Check sheet for the modelled part. Datum: model origin and axes. Units: mm. A direction names the side the tool comes from. Give positions to 0.01 mm unless a question says otherwise; leave off trailing zeros. Write each loop counter-clockwise with the first axis right and the second up, starting at its lowest first coordinate (ties: lowest second). Pieces come first, ordered by that corner, then holes. Notation, with made-up numbers: (29.5, -29.5) -> (70.5, -29.5) arc R16 cw to (70.5, -5.5) -> close; hole circle Ø8 at (36.5, 77.25). An arc over 180 degrees is marked (long way). Use a Markdown table: item, result. Add a question column.
1. Set-up check for faces 4 (the flat face through (24.195, 6, 4)), 5 (the flat face through (30.48, 93, 4)), 6 (the cylindrical face through (46.492, 44.249, 3.757)), 7 (the flat face through (78, 89.408, 4)): record each of +Z, -Z, +X, -X, +Y, -Y from which the full face is reachable in a straight line by a thin tool's end or side.
2. Cross-section at B-B (y = 12.7). Enter the section's corners in (x, z).
3. Scan lines: probe 1 along Z at (x, y) = (7.5, 24); probe 2 along X at (y, z) = (78, 6.5); probe 3 along X at (y, z) = (57.5, 4.75). Record each from-to range of solid material in increasing order. Write a range as [from, to].
4. Cross-section at A-A (x = 17). Enter the section's corners in (y, z).
5. Cross-section at D-D (x = 61). Enter the section's corners in (y, z), then the cut area to 3 significant figures.
6. Release check for a two-part mould opening along Z. For faces 1 (the cylindrical face through (10.454, 12.799, 1.252)), 2 (the flat face through (9, 45, 5.08)), 3 (the flat face through (54, 71, 5.08)) record: released by +Z, released by -Z, zero draft, split by the parting line, or undercut.
7. Gauge pin test, flat ends, axial feed: P1, Ø1.9, axis at y = 93, z = 4, coming from the +X side; P2, Ø3, axis at x = 67.5, y = 88.5, coming from the -Z side; P3, Ø1.9, axis at x = 36.51, y = 89.09, coming from the -Z side. Record the tip position at first contact, or that the pin passes through.
8. Cross-section at C-C (z = 3.75). Count the separate pieces of the cut face and the enclosed holes in it, then the cut area to 3 significant figures.
from build123d import *

# Parameters (mm, degrees)
F0_R     = 2.2479
F0_R_2   = 3.175
F0_R_3   = 11.43
F0_R_4   = 2.8575
F1_DEPTH = 2.54
F2_R     = 2.2479
F2_R_2   = 3.175
F2_R_3   = 2.8575
F2_R_4   = 1.574685516
F3_DEPTH = 2.54
F4_R     = 2.2479
F4_R_2   = 1.574685516
F4_R_3   = 11.4450762602
F5_DEPTH = 2.54
F6_DEPTH = 5.08
F7_W     = 22.86
F7_H     = 2.54
F8_DEPTH = 89.409


with BuildPart() as f1:
    # F0 (on Top) → F1 (new body)
    with BuildSketch(Plane.XY):
        Polygon((0, 89.408), (0, 0), (24.1954457015, 0), (24.1954457015, 11.3160238358), (82.55, 38.608), (82.55, 89.408), (73.66, 89.408), (73.66, 95.758), (30.48, 95.758), (30.48, 89.408), align=None)
        with Locations((12.7, 12.7)):
            Circle(F0_R, mode=Mode.SUBTRACT)
        with Locations((12.7, 44.704)):
            Circle(F0_R, mode=Mode.SUBTRACT)
        with Locations((45.4550236464, 46.2430119514)):
            Circle(F0_R, mode=Mode.SUBTRACT)
        with Locations((36.5125, 57.9755)):
            Circle(F0_R_2, mode=Mode.SUBTRACT)
        with Locations((12.7, 76.708)):
            Circle(F0_R, mode=Mode.SUBTRACT)
        with Locations((36.5125, 89.0905)):
            Circle(F0_R_2, mode=Mode.SUBTRACT)
        with Locations((67.6275, 57.9755)):
            Circle(F0_R_2, mode=Mode.SUBTRACT)
        with Locations((76.7535641789, 48.0743087828)):
            Circle(F0_R, mode=Mode.SUBTRACT)
        with Locations((52.07, 73.533)):
            Circle(F0_R_3, mode=Mode.SUBTRACT)
        with Locations((78.0854150653, 76.0432183743)):
            Circle(F0_R, mode=Mode.SUBTRACT)
        with Locations((67.6275, 89.0905)):
            Circle(F0_R_2, mode=Mode.SUBTRACT)
        with Locations((52.07, 73.533)):
            Circle(F0_R_3)
        with Locations((52.07, 73.533)):
            Circle(F0_R_4, mode=Mode.SUBTRACT)
    extrude(amount=F1_DEPTH)

    # F2 (on face) → F3 (join)
    with BuildSketch(Plane.XY.offset(2.54)):
        Polygon((30.48, 89.408), (25.4, 89.408), (25.4, 11.8793846154), (82.55, 38.608), (82.55, 89.408), (73.66, 89.408), (73.66, 95.758), (30.48, 95.758), align=None)
        with Locations((45.4550236464, 46.2430119514)):
            Circle(F2_R, mode=Mode.SUBTRACT)
        with Locations((36.5125, 57.9755)):
            Circle(F2_R_2, mode=Mode.SUBTRACT)
        with Locations((36.5125, 89.0905)):
            Circle(F2_R_2, mode=Mode.SUBTRACT)
        with Locations((67.6275, 57.9755)):
            Circle(F2_R_2, mode=Mode.SUBTRACT)
        with Locations((76.7535641789, 48.0743087828)):
            Circle(F2_R, mode=Mode.SUBTRACT)
        with Locations((52.07, 73.533)):
            Circle(F2_R_3, mode=Mode.SUBTRACT)
        with Locations((78.0854150653, 76.0432183743)):
            Circle(F2_R, mode=Mode.SUBTRACT)
        with Locations((67.6275, 89.0905)):
            Circle(F2_R_2, mode=Mode.SUBTRACT)
        with Locations((36.5125, 57.9755)):
            Circle(F2_R_2)
        with Locations((36.5125, 57.9755)):
            Circle(F2_R_4, mode=Mode.SUBTRACT)
        with Locations((67.6275, 57.9755)):
            Circle(F2_R_2)
        with Locations((67.6275, 57.9755)):
            Circle(F2_R_4, mode=Mode.SUBTRACT)
        with Locations((67.6275, 89.0905)):
            Circle(F2_R_2)
        with Locations((67.6275, 89.0905)):
            Circle(F2_R_4, mode=Mode.SUBTRACT)
        with Locations((36.5125, 89.0905)):
            Circle(F2_R_2)
        with Locations((36.5125, 89.0905)):
            Circle(F2_R_4, mode=Mode.SUBTRACT)
    extrude(amount=F3_DEPTH)

    # F4 (on face) → F5 (join)
    with BuildSketch(Plane.XY.offset(5.08)):
        Polygon((30.48, 89.408), (25.4, 89.408), (25.4, 11.8793846154), (82.55, 38.608), (82.55, 89.408), (73.66, 89.408), (73.66, 95.758), (30.48, 95.758), align=None)
        with Locations((45.4550236464, 46.2430119514)):
            Circle(F4_R, mode=Mode.SUBTRACT)
        with Locations((36.5125, 57.9755)):
            Circle(F4_R_2, mode=Mode.SUBTRACT)
        with Locations((36.5125, 89.0905)):
            Circle(F4_R_2, mode=Mode.SUBTRACT)
        with Locations((67.6275, 57.9755)):
            Circle(F4_R_2, mode=Mode.SUBTRACT)
        with Locations((76.7535641789, 48.0743087828)):
            Circle(F4_R, mode=Mode.SUBTRACT)
        with Locations((52.07, 73.533)):
            Circle(F4_R_3, mode=Mode.SUBTRACT)
        with Locations((78.0854150653, 76.0432183743)):
            Circle(F4_R, mode=Mode.SUBTRACT)
        with Locations((67.6275, 89.0905)):
            Circle(F4_R_2, mode=Mode.SUBTRACT)
    extrude(amount=F5_DEPTH)

    # F6 (add): a face of the model
    f6_faces = [f1.faces().sort_by_distance(p)[0] for p in [
        (12.7, 88.4785404547, 2.54),
    ]]
    extrude(f6_faces, amount=F6_DEPTH)

    # F7 (on face) → F8 (cut, through all)
    with BuildSketch(Plane(origin=(0, 89.408, 0), x_dir=(-1, 0, 0), z_dir=(0, 1, 0))):
        with Locations((-11.43, 3.81)):
            Rectangle(F7_W, F7_H)
    extrude(amount=-F8_DEPTH, mode=Mode.SUBTRACT)


solid = f1.part
Worked answers:
| question | item | result |
|---|---|---|
| 1 | face 4 | +Z, -Z, +X, -Y |
| 1 | face 5 | +Z, -Z, -X, +Y |
| 1 | face 6 | +Z, -Z |
| 1 | face 7 | +Z, -Z, +X, +Y |
| 2 | outline | (0, 0) -> (10.45, 0) -> (10.45, 2.54) -> (0, 2.54) -> close; (0, 5.08) -> (10.45, 5.08) -> (10.45, 7.62) -> (0, 7.62) -> close; (14.95, 0) -> (27.15, 0) -> (27.15, 7.62) -> (14.95, 7.62) -> (14.95, 5.08) -> (22.86, 5.08) -> (22.86, 2.54) -> (14.95, 2.54) -> close |
| 3 | probe 1 | z = [0, 2.54], [5.08, 7.62] |
| 3 | probe 2 | x = [0, 10.86], [14.54, 41.53], [62.61, 76.98], [79.19, 82.55] |
| 3 | probe 3 | x = [22.86, 35.01], [38.01, 66.13], [69.13, 82.55] |
| 4 | outline | (0, 0) -> (89.41, 0) -> (89.41, 2.54) -> (0, 2.54) -> close; (0, 5.08) -> (89.41, 5.08) -> (89.41, 7.62) -> (0, 7.62) -> close |
| 5 | outline | (28.53, 0) -> (95.76, 0) -> (95.76, 7.62) -> (80.69, 7.62) -> (80.69, 5.08) -> (66.37, 5.08) -> (66.37, 7.62) -> (28.53, 7.62) -> close |
| 5 | area | 476 mm² |
| 6 | face 1 | zero draft |
| 6 | face 2 | undercut |
| 6 | face 3 | released by +Z |
| 7 | P1 | stops at x = 73.66 |
| 7 | P2 | stops at z = 2.54 |
| 7 | P3 | passes through |
| 8 | separate pieces | 1 |
| 8 | enclosed holes | 8 |
| 8 | area | 4,050 mm² |
